Check sheet for the modelled part. Datum: model origin and axes. Units: mm. Give positions to 0.01 mm unless a question says otherwise; leave off trailing zeros. Loops run counter-clockwise (first coordinate to the right, second up) from the corner with the lowest first, then second, coordinate; pieces in that order, holes last. Notation, with made-up numbers: (8, 58) -> (21, 58) arc R16 ccw to (21, 88) -> close; hole circle Ø8 at (74.5, 64). An arc over 180 degrees is marked (long way). Write each question's results on one line, items separated by ' | '. Start each with the question number.
1. Cross-section at A-A on z = -0.8. Record the boundary of the cut face in (x, y), and give its area (3 significant figures).
2. Mould release check, pull along X, two halves, no side actions. Record for faces 1 (the face through (0, 11, 0)), 2 (the face through (-6.5, 5, 0)), 3 (the face through (0, 0.5, 0)): +X half, -X half, draft (parallel to the pull), parting line (faces both ways), or undercut.
3. Cross-section at D-D on z = 1.6. Record the boundary of the cut face in (x, y), and give its area (3 significant figures).
4. Material ranges on L1, parallel to Y at x = 2.75, z = 0.45; L2, parallel to Z at x = 2.75, y = 9; L3, parallel to Y at x = 5.75, z = 2.1, recorded low to high. Write a range as from..to.
5. Cross-section at C-C on x = 5.5. Record the boundary of the cut face in (y, z), and give its area (3 significant figures).
6. Cross-section at B-B on y = 1. Record the boundary of the cut face in (x, z).
7. Gauge pin test, flat ends, axial feed: pin 1 Ø3 at (x, y) = (-0.5, 7.5) entering from -Z; pin 2 Ø2.5 at (x, z) = (-0.5, 0.5) entering from -Y. Record the tip position at first contact, or that the pin passes through.
from build123d import *

# Parameters (mm, degrees)
SKETCH1_W           = 13
SKETCH1_H           = 5
BOSS_EXTRUDE1_DEPTH = 11
CUT_EXTRUDE1_DEPTH  = 6
FILLET1_R           = 0.2
SKETCH3_R           = 0.3


with BuildPart() as part:
    # Sketch1 → Boss-Extrude1 (new body)
    with BuildSketch(Plane(origin=(0, 0, 0), x_dir=(1, 0, 0), z_dir=(0, 1, 0))):
        Rectangle(SKETCH1_W, SKETCH1_H)
    extrude(amount=BOSS_EXTRUDE1_DEPTH)

    # Sketch2 → Cut-Extrude1 (cut, through all)
    with BuildSketch(Plane.XY.offset(2.5)):
        Polygon((-4.5, 0), (-4, 0.5), (4, 0.5), (4.5, 0), (4.5, -1.5), (-4.5, -1.5), align=None)
    extrude(amount=-CUT_EXTRUDE1_DEPTH, mode=Mode.SUBTRACT)

    # Fillet1
    fillet1_edges = [part.edges().sort_by_distance(p)[0] for p in [
        (6.5, 11, 0),
        (0, 11, -2.5),
        (-5.5, 0, -2.5),
        (5.5, 0, 2.5),
        (4.25, 0.25, 2.5),
        (0, 0.5, 2.5),
        (-4.25, 0.25, 2.5),
        (-4.25, 0.25, -2.5),
        (-4.5, 0, 0),
        (0, 0.5, -2.5),
        (-4, 0.5, 0),
        (4.25, 0.25, -2.5),
        (4, 0.5, 0),
        (4.5, 0, 0),
        (-6.5, 11, 0),
        (5.5, 0, -2.5),
        (6.5, 0, 0),
        (-5.5, 0, 2.5),
        (-6.5, 0, 0),
        (0, 11, 2.5),
        (-6.5, 5.5, -2.5),
        (6.5, 5.5, -2.5),
        (6.5, 5.5, 2.5),
        (-6.5, 5.5, 2.5),
    ]]
    fillet(fillet1_edges, radius=FILLET1_R)

    # Sweep1: sweep along a path in Sketch5
    with BuildLine(Plane(origin=(-5, 0, 0), x_dir=(0, 0, -1), z_dir=(1, 0, 0))) as sweep1_path:
        Line((0, 0), (0, -0.1))
        ThreePointArc((0, -0.1), (0.146446609, -0.453553391), (0.5, -0.6))
        Line((0.5, -0.6), (3, -0.6))
    # Sketch3 → Sweep1 (sweep)
    with BuildSketch(Plane.XZ):
        with Locations((-5, 0)):
            Circle(SKETCH3_R)
    sweep1 = sweep(path=sweep1_path.line)

    # Mirror1: Sweep1 across plane
    add(sweep1.mirror(Plane(origin=(0, 0, 0), x_dir=(0, 0, 1), z_dir=(1, 0, 0))))


solid = part.part
Geometry says:
1) outline: (-6.5, 0.2) arc R0.2 ccw to (-6.3, 0) -> (-4.58, 0) arc R0.2 ccw to (-4.44, 0.06) -> (-4.06, 0.44) arc R0.2 cw to (-3.92, 0.5) -> (3.92, 0.5) arc R0.2 cw to (4.06, 0.44) -> (4.44, 0.06) arc R0.2 ccw to (4.58, 0) -> (6.3, 0) arc R0.2 ccw to (6.5, 0.2) -> (6.5, 10.8) arc R0.2 ccw to (6.3, 11) -> (-6.3, 11) arc R0.2 ccw to (-6.5, 10.8) -> close; circle Ø0.6 at (-5, -0.6); circle Ø0.6 at (5, -0.6) | area: 139 mm^2
2) face 1: draft | face 2: -X half | face 3: undercut
3) outline: (-6.5, 0.2) arc R0.2 ccw to (-6.3, 0) -> (-4.58, 0) arc R0.2 ccw to (-4.44, 0.06) -> (-4.06, 0.44) arc R0.2 cw to (-3.92, 0.5) -> (3.92, 0.5) arc R0.2 cw to (4.06, 0.44) -> (4.44, 0.06) arc R0.2 ccw to (4.58, 0) -> (6.3, 0) arc R0.2 ccw to (6.5, 0.2) -> (6.5, 10.8) arc R0.2 ccw to (6.3, 11) -> (-6.3, 11) arc R0.2 ccw to (-6.5, 10.8) -> close | area: 139 mm^2
4) L1: 0.5..11 | L2: -2.5..2.5 | L3: 0..11
5) outline: (0, -2.3) arc R0.2 ccw to (0.2, -2.5) -> (10.8, -2.5) arc R0.2 ccw to (11, -2.3) -> (11, 2.3) arc R0.2 ccw to (10.8, 2.5) -> (0.2, 2.5) arc R0.2 ccw to (0, 2.3) -> close | area: 55.0 mm^2
6) outline: (-6.5, -2.3) arc R0.2 ccw to (-6.3, -2.5) -> (6.3, -2.5) arc R0.2 ccw to (6.5, -2.3) -> (6.5, 2.3) arc R0.2 ccw to (6.3, 2.5) -> (-6.3, 2.5) arc R0.2 ccw to (-6.5, 2.3) -> close
7) pin 1: z = -2.5 | pin 2: y = 0.5
